from build123d import *

# Parameters (mm, degrees)
SKETCH1_R               = 2.1
SKETCH1_R_2             = 1.6
BOSS_EXTRUDE1_DEPTH     = 10
CUT_EXTRUDE1_DEPTH      = 8
SKETCH3_W               = 12
SKETCH3_H               = 6
CUT_EXTRUDE2_DEPTH      = 35.369317712
CIRPATTERN1_COUNT       = 4
FILLET1_R               = 1
CUT_EXTRUDE3_DEPTH      = 25.093567606
CUT_EXTRUDE3_DEPTH_BACK = 25.093567606
SKETCH4_W               = 64.927368138
SKETCH4_H               = 2
FILLET2_R               = 1.5


# Some blends are built 0.0001 mm under size
with BuildPart() as part:
    # Sketch1 → Boss-Extrude1 (new body)
    with BuildSketch(Plane(origin=(0, 0, 0), x_dir=(1, 0, 0), z_dir=(0, 1, 0))):
        with BuildLine():
            Line((-12.5, -15.5), (12.5, -15.5))
            ThreePointArc((12.5, -15.5), (14.621320344, -14.621320344), (15.5, -12.5))
            Line((15.5, -12.5), (15.5, 12.5))
            ThreePointArc((15.5, 12.5), (14.621320344, 14.621320344), (12.5, 15.5))
            Line((12.5, 15.5), (-12.5, 15.5))
            ThreePointArc((-12.5, 15.5), (-14.621320344, 14.621320344), (-15.5, 12.5))
            Line((-15.5, 12.5), (-15.5, -12.5))
            ThreePointArc((-15.5, -12.5), (-14.621320344, -14.621320344), (-12.5, -15.5))
        make_face()
        with Locations(Location((0, 0, 0), (0, 0, 270))):
            Circle(SKETCH1_R, mode=Mode.SUBTRACT)
        with Locations(Location((-8.5, 8.5, 0), (0, 0, 270))):
            Circle(SKETCH1_R_2, mode=Mode.SUBTRACT)
        with Locations(Location((8.5, 8.5, 0), (0, 0, 270))):
            Circle(SKETCH1_R_2, mode=Mode.SUBTRACT)
        with Locations(Location((8.5, -8.5, 0), (0, 0, 270))):
            Circle(SKETCH1_R_2, mode=Mode.SUBTRACT)
        with Locations(Location((-8.5, -8.5, 0), (0, 0, 270))):
            Circle(SKETCH1_R_2, mode=Mode.SUBTRACT)
    extrude(amount=BOSS_EXTRUDE1_DEPTH)

    # Sketch2 → Cut-Extrude1 (cut)
    with BuildSketch(Plane(origin=(0, 10, 0), x_dir=(1, 0, 0), z_dir=(0, 1, 0))):
        with BuildLine():
            Line((-12.5, -13.5), (12.5, -13.5))
            ThreePointArc((12.5, -13.5), (13.207106781, -13.207106781), (13.5, -12.5))
            Line((13.5, -12.5), (13.5, 12.5))
            ThreePointArc((13.5, 12.5), (13.207106781, 13.207106781), (12.5, 13.5))
            Line((12.5, 13.5), (-12.5, 13.5))
            ThreePointArc((-12.5, 13.5), (-13.207106781, 13.207106781), (-13.5, 12.5))
            Line((-13.5, 12.5), (-13.5, -12.5))
            ThreePointArc((-13.5, -12.5), (-13.207106781, -13.207106781), (-12.5, -13.5))
        make_face()
    extrude(amount=-CUT_EXTRUDE1_DEPTH, mode=Mode.SUBTRACT)

    # Sketch3 → Cut-Extrude2 (cut, through all)
    with BuildSketch(Plane.XY.offset(-13.5)):
        with Locations((0, 6)):
            Rectangle(SKETCH3_W, SKETCH3_H)
    cut_extrude2 = extrude(amount=-CUT_EXTRUDE2_DEPTH, mode=Mode.SUBTRACT)

    # CirPattern1: Cut-Extrude2 ×4 about axis
    cirpattern1_axis = Axis((0, 0, 0), (0, 1, 0))
    for i in range(1, CIRPATTERN1_COUNT):
        add(cut_extrude2.rotate(cirpattern1_axis, i * 360 / CIRPATTERN1_COUNT), mode=Mode.SUBTRACT)

    # Fillet1
    fillet1_edges = [part.edges().sort_by_distance(p)[0] for p in [
        (-15.5, 6, 6),
        (-14.5, 3, 6),
        (-15.5, 9, 0),
        (-14.5, 9, 6),
        (-15.5, 6, -6),
        (-14.5, 9, -6),
        (-15.5, 3, 0),
        (-14.5, 3, -6),
        (6, 6, 15.5),
        (6, 3, 14.5),
        (0, 9, 15.5),
        (6, 9, 14.5),
        (-6, 6, 15.5),
        (-6, 9, 14.5),
        (0, 3, 15.5),
        (-6, 3, 14.5),
        (15.5, 6, -6),
        (14.5, 3, -6),
        (15.5, 9, 0),
        (14.5, 9, -6),
        (15.5, 6, 6),
        (14.5, 9, 6),
        (15.5, 3, 0),
        (14.5, 3, 6),
        (-6, 6, -15.5),
        (-6, 3, -14.5),
        (0, 9, -15.5),
        (-6, 9, -14.5),
        (6, 6, -15.5),
        (6, 9, -14.5),
        (0, 3, -15.5),
        (6, 3, -14.5),
    ]]
    fillet(fillet1_edges, radius=FILLET1_R - 0.0001)  # a hair under: the kernel refuses the full size

    # Sketch4 → Cut-Extrude3 (cut, two sides: drawn at the far end of the back side and taken through both)
    with BuildSketch(Plane(origin=(0, 0, 0), x_dir=(0, 0, -1), z_dir=(1, 0, 0)).offset(-CUT_EXTRUDE3_DEPTH_BACK)):
        with Locations((2.454919732, 9)):
            Rectangle(SKETCH4_W, SKETCH4_H)
    extrude(amount=CUT_EXTRUDE3_DEPTH + CUT_EXTRUDE3_DEPTH_BACK, mode=Mode.SUBTRACT)

    # Fillet2
    # the kernel refuses this fillet: 1.5 mm, written as the material it takes off along each edge
    with BuildSketch(Plane(origin=(12.5, 8, -12.5), x_dir=(0, 0, -1), z_dir=(-1, 0, 0))) as fillet2_piece_1:
        with BuildLine():
            CenterArc((3 - FILLET2_R, FILLET2_R), FILLET2_R, 270, 90)
            Line((3 - FILLET2_R, 0), (3, 0))
            Line((3, 0), (3, FILLET2_R))
        make_face()
    revolve(axis=Axis((12.5, 8, -12.5), (0, -1, 0)), revolution_arc=90, mode=Mode.SUBTRACT)
    with BuildSketch(Plane(origin=(3.2499, 8, -15.5), x_dir=(0, -1, 0), z_dir=(1, 0, 0)), Plane(origin=(15.5, 8, -12.5), x_dir=(0, -1, 0), z_dir=(0, 0, 1)), Plane(origin=(15.5, 8, 3.2499), x_dir=(0, -1, 0), z_dir=(0, 0, 1)), Plane(origin=(12.5, 8, 15.5), x_dir=(0, -1, 0), z_dir=(-1, 0, 0)), Plane(origin=(-15.5, 8, 12.5), x_dir=(0, -1, 0), z_dir=(0, 0, -1)), Plane(origin=(-15.5, 8, -3.2499), x_dir=(0, -1, 0), z_dir=(0, 0, -1))) as fillet2_piece_2:
        with BuildLine():
            CenterArc((FILLET2_R, -FILLET2_R), FILLET2_R, 90, 90)
            Line((0, -FILLET2_R), (0, 0))
            Line((0, 0), (FILLET2_R, 0))
        make_face()
    extrude(amount=9.2501, mode=Mode.SUBTRACT)
    with BuildSketch(Plane(origin=(12.5, 8, 12.5), x_dir=(1, 0, 0), z_dir=(0, 0, -1))) as fillet2_piece_3:
        with BuildLine():
            CenterArc((3 - FILLET2_R, FILLET2_R), FILLET2_R, 270, 90)
            Line((3 - FILLET2_R, 0), (3, 0))
            Line((3, 0), (3, FILLET2_R))
        make_face()
    revolve(axis=Axis((12.5, 8, 12.5), (0, -1, 0)), revolution_arc=90, mode=Mode.SUBTRACT)
    with BuildSketch(Plane(origin=(-3.2499, 8, 15.5), x_dir=(0, 0, -1), z_dir=(-1, 0, 0)), Plane(origin=(-12.5, 8, -15.5), x_dir=(0, 0, 1), z_dir=(1, 0, 0))) as fillet2_piece_4:
        with BuildLine():
            CenterArc((FILLET2_R, FILLET2_R), FILLET2_R, 180, 90)
            Line((0, FILLET2_R), (0, 0))
            Line((0, 0), (FILLET2_R, 0))
        make_face()
    extrude(amount=9.2501, mode=Mode.SUBTRACT)
    with BuildSketch(Plane(origin=(-12.5, 8, 12.5), x_dir=(0, 0, 1), z_dir=(1, 0, 0))) as fillet2_piece_5:
        with BuildLine():
            CenterArc((3 - FILLET2_R, FILLET2_R), FILLET2_R, 270, 90)
            Line((3 - FILLET2_R, 0), (3, 0))
            Line((3, 0), (3, FILLET2_R))
        make_face()
    revolve(axis=Axis((-12.5, 8, 12.5), (0, -1, 0)), revolution_arc=90, mode=Mode.SUBTRACT)
    with BuildSketch(Plane(origin=(-12.5, 8, -12.5), x_dir=(-1, 0, 0), z_dir=(0, 0, 1))) as fillet2_piece_6:
        with BuildLine():
            CenterArc((3 - FILLET2_R, FILLET2_R), FILLET2_R, 270, 90)
            Line((3, FILLET2_R), (3, 0))
            Line((3, 0), (3 - FILLET2_R, 0))
        make_face()
    revolve(axis=Axis((-12.5, 8, -12.5), (0, -1, 0)), revolution_arc=90, mode=Mode.SUBTRACT)


solid = part.part
Source: CAD feature listing. Evaluate the final solid. Frame: model axes, mm. A direction names the side the tool comes from. Give positions to 0.01 mm unless a question says otherwise; leave off trailing zeros. Loops run counter-clockwise (first coordinate to the right, second up) from the corner with the lowest first, then second, coordinate; pieces in that order, holes last. Notation, with made-up numbers: (-25.5, 65.25) -> (22.5, 65.25) arc R28 ccw to (22.5, 92.25) -> close; hole circle Ø2 at (-32, 21). An arc over 180 degrees is marked (long way). Use a Markdown table: item, result. Add a question column.
1) Line query: line 1 along X through (y, z) = (1.3, 8.5); line 2 along X through (y, z) = (4, 7.5). Output: solid intervals per line, ascending. Write a range as [from, to].
2) Section query C-C, the plane y = 1.5. Return the cut outline in (x, z).
3) First-contact query: pin 1 (5 mm diameter, centred on x = -8.5, z = -8.5, fed in from -Y); pin 2 (2 mm diameter, centred on x = 9.5, z = -5.5, fed in from +Y); pin 3 (1.1 mm diameter, centred on x = -14, y = 5.5, fed in from -Z); pin 4 (0.5 mm diameter, centred on x = -14, y = 6.5, fed in from +Z). Flat tips, straight axial feed; report the tip coordinate or a pass-through.
4) Section query D-D, the plane x = 0. Return the cut outline in (y, z), then the cut area to 3 significant figures.
5) Section query A-A, the plane x = -8.5. Return the cut outline in (y, z), then the cut area to 3 significant figures.
6) Reachability of faces 1 (the face through (0, 3, 14)), 2 (the face through (6.301, 5.55, 15.215)), 3 (the face through (15.215, 2.699, 0.07)) from +Z, -Z, +X, -X, +Y, -Y: full face, straight path, thin tool, end or side. Return the list, or none.
7) Pull-direction query (Z, two-part tool) for faces 4 (the face through (5.699, 3.285, 14.007)), 5 (the face through (13.215, 5.042, -13.199)), 6 (the face through (-14, 3, 0)), 7 (the face through (-14.6, 3.2, -14.64)); classes: +Z half, -Z half, draft (parallel to the pull), parting line (faces both ways), or undercut.
8) Section query B-B, the plane z = 0. Return the cut outline in (x, y).
Numbers:
| question | item | result |
|---|---|---|
| 1 | line 1 | x = [-15.5, -10.1], [-6.9, 6.9], [10.1, 15.5] |
| 1 | line 2 | x = [-15.5, -13.5], [13.5, 15.5] |
| 2 | outline | (-15.5, -12.5) arc R3 ccw to (-12.5, -15.5) -> (12.5, -15.5) arc R3 ccw to (15.5, -12.5) -> (15.5, 12.5) arc R3 ccw to (12.5, 15.5) -> (-12.5, 15.5) arc R3 ccw to (-15.5, 12.5) -> close; hole circle Ø3.2 at (-8.5, -8.5); hole circle Ø3.2 at (-8.5, 8.5); hole circle Ø4.2 at (0, 0); hole circle Ø3.2 at (8.5, -8.5); hole circle Ø3.2 at (8.5, 8.5) |
| 3 | pin 1 | stops at y = 0 |
| 3 | pin 2 | stops at y = 2 |
| 3 | pin 3 | stops at z = -15.35 |
| 3 | pin 4 | stops at z = 15.23 |
| 4 | outline | (0, -15.5) -> (2, -15.5) arc R1 ccw to (3, -14.5) -> (3, -13.5) -> (2, -13.5) -> (2, -2.1) -> (0, -2.1) -> close; (0, 2.1) -> (2, 2.1) -> (2, 13.5) -> (3, 13.5) -> (3, 14.5) arc R1 ccw to (2, 15.5) -> (0, 15.5) -> close |
| 4 | area | 57.2 mm2 |
| 5 | outline | (0, -15.5) -> (6.5, -15.5) arc R1.5 ccw to (8, -14) -> (8, -13.5) -> (2, -13.5) -> (2, -10.1) -> (0, -10.1) -> close; (0, -6.9) -> (2, -6.9) -> (2, 6.9) -> (0, 6.9) -> close; (0, 10.1) -> (2, 10.1) -> (2, 13.5) -> (8, 13.5) -> (8, 14) arc R1.5 ccw to (6.5, 15.5) -> (0, 15.5) -> close |
| 5 | area | 72.2 mm2 |
| 6 | face 1 | +Z, -Z, +Y |
| 6 | face 2 | +Z, +Y |
| 6 | face 3 | +X, +Y |
| 7 | face 4 | draft |
| 7 | face 5 | undercut |
| 7 | face 6 | undercut |
| 7 | face 7 | -Z half |
| 8 | outline | (-15.5, 0) -> (-2.1, 0) -> (-2.1, 2) -> (-13.5, 2) -> (-13.5, 3) -> (-14.5, 3) arc R1 ccw to (-15.5, 2) -> close; (2.1, 0) -> (15.5, 0) -> (15.5, 2) arc R1 ccw to (14.5, 3) -> (13.5, 3) -> (13.5, 2) -> (2.1, 2) -> close |
